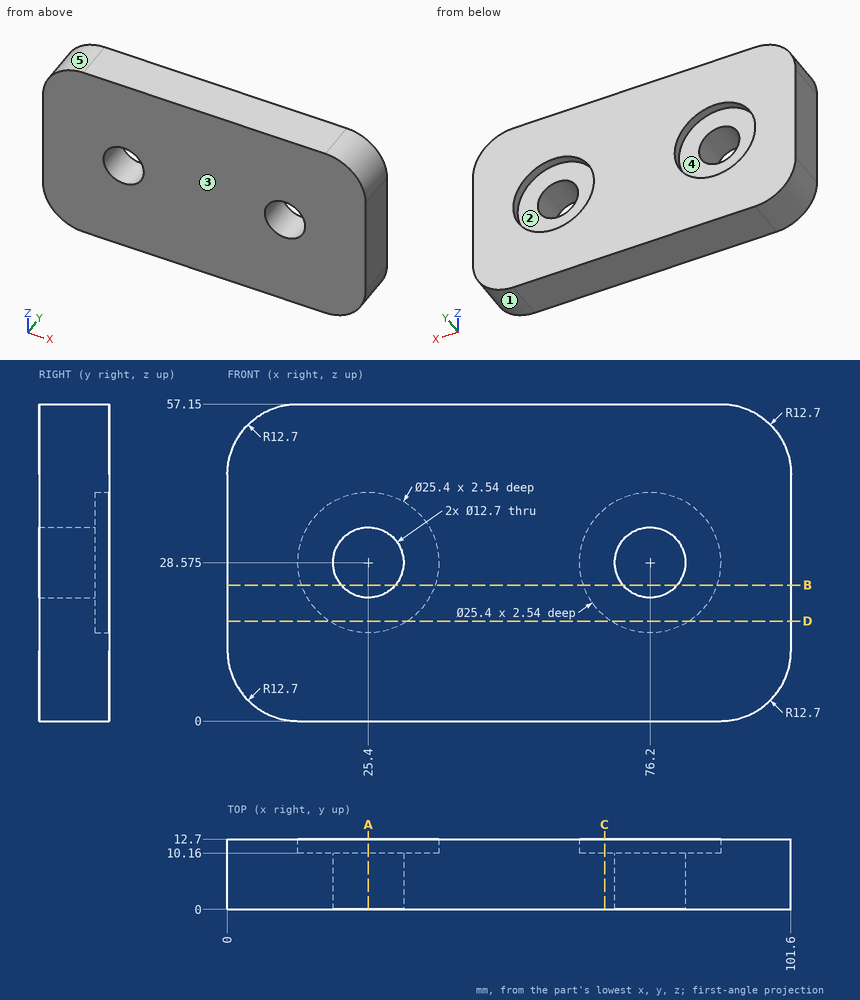
Design review of the part shown in the three views and the two pictorial views. Dimensions are in mm from the part's minimum x, y and z. A direction names the side the tool comes from. Coordinates: 2 decimals unless noted, no trailing zeros. Order: outer loops, then holes, each group sorted by start corner. A loop starts at its lowest first (then second) coordinate and runs counter-clockwise, first axis right, second up. Notation, with made-up numbers: (5, 89.25) -> (12, 89.25) arc R23 cw to (12, 103.25) -> close; hole circle Ø1 at (-3.75, -6.75). An arc over 180 degrees is marked (long way). Use one line per item in the form item = value. Start each with the question number.
(1) For the marked faces 4 and 5, list the 3-axis set-ups (+Z, -Z, +X, -X, +Y, -Y) from which the entire face can be reached by the end or side of a thin tool; tool diameter is ignored.
(2) Add section B-B on z = 24.5. State the section outline as (x, y) points, plus the area to 3 significant figures.
(3) The part is to be moulded in two halves that separate along X. For the marked faces 1, 2 and 3, say which applies: +X half, -X half, draft (parallel to the pull), parting line (faces both ways), or undercut.
(4) Insertion check: pin 1 (1.5 mm diameter, centred on y = 6.5, z = 14, fed in from -X); pin 2 (16.5 mm diameter, centred on x = 76.2, z = 28.575, fed in from +Y). Each pin has a flat end and moves straight along its axis. Give the tip position at first contact, or say it passes through.
(5) Add section D-D on z = 18. State the section outline as (x, y) points, plus the area to 3 significant figures.
(6) Add section C-C on x = 68. State the section outline as (y, z) points, plus the area to 3 significant figures.
(7) For probe 1 along Z at (x, y) = (25.4, 5.5) (3 decimals); probe 2 along X at (y, z) = (11, 33); probe 3 along X at (y, z) = (7, 33), list the stretches that pass through material, from the lowest coordinate up.
(8) Add section A-A on x = 25.4. State the section outline as (y, z) points (3 decimals), plus the area to 3 significant figures.
Answer block:
q1.face_4 = +Y
q1.face_5 = +Z, -X, +Y, -Y
q2.outline = (0, 0) -> (20.53, 0) -> (20.53, 10.16) -> (13.37, 10.16) -> (13.37, 12.7) -> (0, 12.7) -> close; (30.27, 0) -> (71.33, 0) -> (71.33, 10.16) -> (64.17, 10.16) -> (64.17, 12.7) -> (37.43, 12.7) -> (37.43, 10.16) -> (30.27, 10.16) -> close; (81.07, 0) -> (101.6, 0) -> (101.6, 12.7) -> (88.23, 12.7) -> (88.23, 10.16) -> (81.07, 10.16) -> close
q2.area = 970 mm²
q3.face_1 = +X half
q3.face_2 = undercut
q3.face_3 = draft
q4.pin_1 = 0
q4.pin_2 = 10.16
q5.outline = (0, 0) -> (101.6, 0) -> (101.6, 12.7) -> (83.23, 12.7) -> (83.23, 10.16) -> (69.17, 10.16) -> (69.17, 12.7) -> (32.43, 12.7) -> (32.43, 10.16) -> (18.37, 10.16) -> (18.37, 12.7) -> (0, 12.7) -> close
q5.area = 1,220 mm²
q6.outline = (0, 0) -> (12.7, 0) -> (12.7, 18.88) -> (10.16, 18.88) -> (10.16, 38.27) -> (12.7, 38.27) -> (12.7, 57.15) -> (0, 57.15) -> close
q6.area = 677 mm²
q7.probe_1 = 0 to 22.225, 34.925 to 57.15
q7.probe_2 = 0 to 13.5, 37.3 to 64.3, 88.1 to 101.6
q7.probe_3 = 0 to 20.85, 29.95 to 71.65, 80.75 to 101.6
q8.outline = (0, 0) -> (12.7, 0) -> (12.7, 15.875) -> (10.16, 15.875) -> (10.16, 22.225) -> (0, 22.225) -> close; (0, 34.925) -> (10.16, 34.925) -> (10.16, 41.275) -> (12.7, 41.275) -> (12.7, 57.15) -> (0, 57.15) -> close
q8.area = 532 mm²
